CAD build for the part. Positions are in the model's coordinates, mm. Face numbers are marked on the shaded views. A direction names the side the tool comes from. Round coordinates to 2 decimals unless told otherwise and drop trailing zeros. Write each loop counter-clockwise with the first axis right and the second up, starting at its lowest first coordinate (ties: lowest second). Pieces come first, ordered by that corner, then holes. Notation, with made-up numbers: (-21.75, 78) - (20.25, 78) arc R21 ccw to (20.25, 101) - close; hole circle Ø8 at (63.5, 17.25). An arc over 180 degrees is marked (long way). Use one line per item in the form item = value. Start each with the question number.
Item 1: Tool access for the marked faces 4, 5 and 6: list every direction of +Z, -Z, +X, -X, +Y, -Y with a clear straight run to the whole face (end or side of a thin tool).
Item 2: Band-saw the part on A-A, the plane z = 0. List the corners of the cut face in (x, y), and give its area (4 significant figures).
Item 3: Pull direction Z, two halves, no side cores. Call the marked faces 1, 2 and 3: +Z half, -Z half, draft (parallel to the pull), parting line (faces both ways), or undercut.
Item 4: Band-saw the part on B-B, the plane x = 0. List the corners of the cut face in (y, z).
Item 5: Pin check, flat tips, straight feed: pin 1 (1 mm diameter, centred on y = -20.5, z = 2, fed in from +X); pin 2 (6 mm diameter, centred on x = -4, y = -10, fed in from -Z); pin 3 (4 mm diameter, centred on x = 5.5, y = -15.5, fed in from +Z). Stop position of each tip, or through.
Item 6: Band-saw the part on D-D, the plane z = -4. List the corners of the cut face in (x, y).
Item 7: Drill centre lines: L1, parallel to Y at x = 0, z = -5.25; L2, parallel to Y at x = -4, z = -1; L3, parallel to Z at x = 1.75, y = -1.5. Where is each one in solid material? Low to high.
Item 8: Band-saw the part on C-C, the plane y = -16. List the corners of the cut face in (x, z), and give its area (3 significant figures).
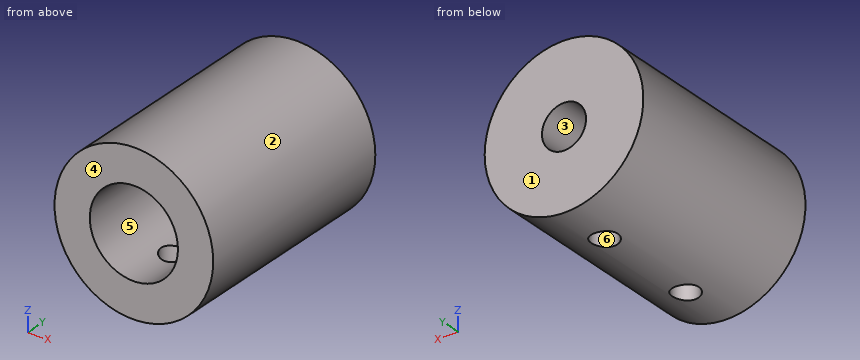
from build123d import *

# Parameters (mm, degrees)
F0_R     = 9
F1_DEPTH = 25
F2_R     = 5
F3_DEPTH = 12.5
F4_R     = 2.5
F5_DEPTH = 12.5
F6_R     = 1.5
F7_DEPTH = 25


with BuildPart() as f1:
    # F0 (on Front) → F1 (new body)
    with BuildSketch(Plane.XZ):
        Circle(F0_R)
    extrude(amount=F1_DEPTH)

    # F2 (on face) → F3 (cut)
    with BuildSketch(Plane.XZ.offset(25)):
        Circle(F2_R)
    extrude(amount=-F3_DEPTH, mode=Mode.SUBTRACT)

    # F4 (on face) → F5 (cut)
    with BuildSketch(Plane(origin=(0, 0, 0), x_dir=(-1, 0, 0), z_dir=(0, 1, 0))):
        Circle(F4_R)
    extrude(amount=-F5_DEPTH, mode=Mode.SUBTRACT)

    # F6 (on Top) → F7 (cut)
    with BuildSketch(Plane.XY):
        with Locations((0, -6.25)):
            Circle(F6_R)
        with Locations((0, -18.75)):
            Circle(F6_R)
    extrude(amount=-F7_DEPTH, mode=Mode.SUBTRACT)


solid = f1.part
Determined:
q1.face_4 = +Z, -Z, +X, -X, -Y
q1.face_5 = -Y
q1.face_6 = -Z
q2.outline = (-9, -25) - (-5, -25) - (-5, -12.5) - (-2.5, -12.5) - (-2.5, 0) - (-9, 0) - close; (2.5, -12.5) - (5, -12.5) - (5, -25) - (9, -25) - (9, 0) - (2.5, 0) - close
q2.area = 262.5 mm²
q3.face_1 = draft
q3.face_2 = parting line
q3.face_3 = undercut
q4.outline = (-25, -9) - (-20.25, -9) - (-20.25, -5) - (-25, -5) - close; (-25, 5) - (-12.5, 5) - (-12.5, 2.5) - (0, 2.5) - (0, 9) - (-25, 9) - close; (-17.25, -9) - (-7.75, -9) - (-7.75, -2.5) - (-12.5, -2.5) - (-12.5, -5) - (-17.25, -5) - close; (-4.75, -9) - (0, -9) - (0, -2.5) - (-4.75, -2.5) - close
q5.pin_1 = 8.87
q5.pin_2 = -8.94
q5.pin_3 = 8.29
q6.outline = (-8.06, -25) - (-3, -25) - (-3, -12.5) - (3, -12.5) - (3, -25) - (8.06, -25) - (8.06, 0) - (-8.06, 0) - close; hole circle Ø3 at (0, -6.25)
q7.L1 = -25 to -20.25, -17.25 to -7.75, -4.75 to 0
q7.L2 = -12.5 to 0
q7.L3 = -8.83 to -1.79, 1.79 to 8.83
q8.outline = circle Ø18 at (0, 0); hole circle Ø10 at (0, 0)
q8.area = 176 mm²
